Input: dimensioned drawing with shaded views. Units: mm. Origin: part minimum x, y, z. Give positions to 0.01 mm unless a question says otherwise; leave off trailing zeros. Order: outer loops, then holes, each group sorted by start corner. A loop starts at its lowest first (then second) coordinate and runs counter-clockwise, first axis right, second up. Notation, with made-up numbers: (22.5, 11) -> (79.5, 11) arc R15 ccw to (79.5, 15) -> close; hole circle Ø10 at (62.25, 55). An arc over 180 degrees is marked (long way). Use CSV: the item, a comma, the result in double quotes.
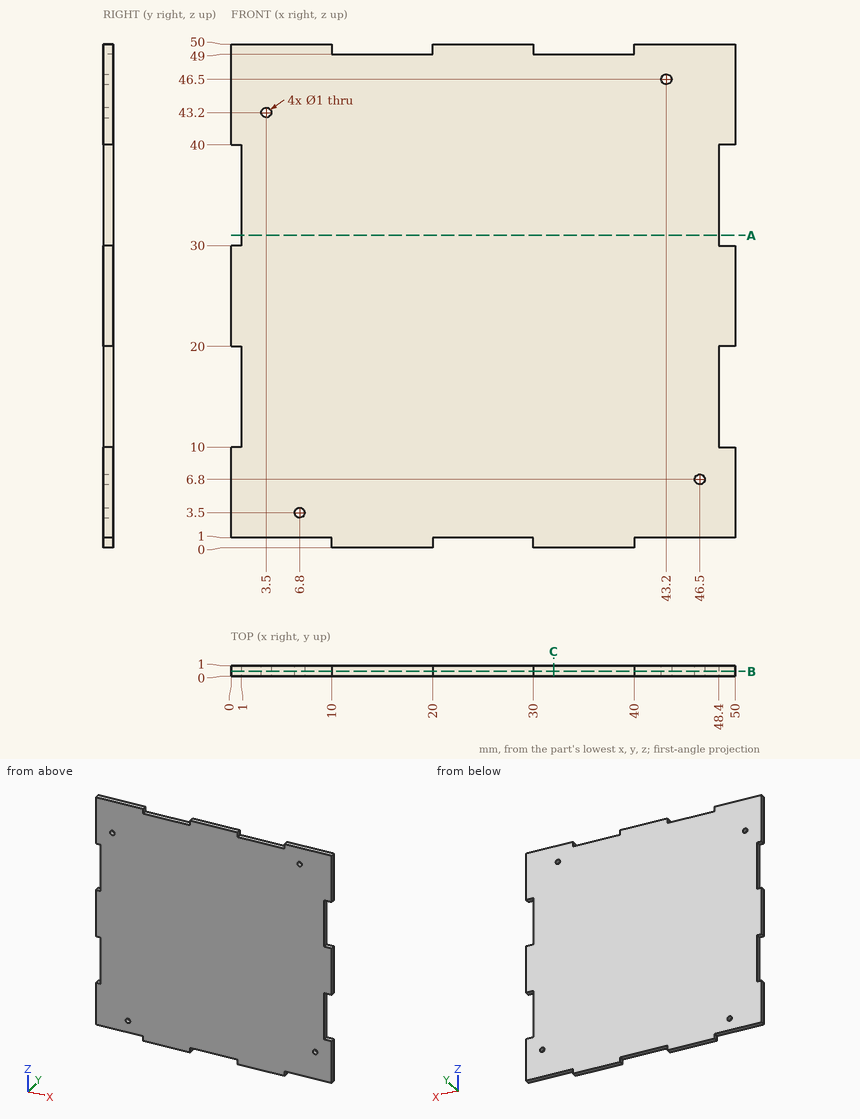
1. Section query A-A on z = 31. Return loops of the section in (x, y), plus the area to 3 significant figures.
Answer below:
outline,"(1, 0) -> (48.4, 0) -> (48.4, 1) -> (1, 1) -> close"
area,"47.4 mm²"
2. Section query B-B on y = 0.45. Count the separate pieces of the cut face and the enclosed holes in it, plus the area to 3 significant figures.
Answer below:
separate pieces,"1"
enclosed holes,"4"
area,"2,390 mm²"
3. Section query C-C on x = 32. Return loops of the section in (y, z).
Answer below:
outline,"(0, 0) -> (1, 0) -> (1, 49) -> (0, 49) -> close"
4. Pin query (flat end, axial travel): P1, Ø0.5, axis at x = 6.5, y = 0.5, coming from the -Z side; P2, Ø0.5, axis at y = 0.5, z = 0.5, coming from the -X side. Return the tip coordinate at first contact, or that it passes through.
Answer below:
P1,"stops at z = 1"
P2,"stops at x = 10"
5. Ray query, line 1 along Z through (x, y) = (43.2, 0.6); line 2 along Z through (x, y) = (46.5, 0.4); line 3 along X through (y, z) = (0.6, 3.5). Return the intervals inside material, ascending.
Answer below:
line 1,"z = 1 to 46, 47 to 50"
line 2,"z = 1 to 6.3, 7.3 to 50"
line 3,"x = 0 to 6.3, 7.3 to 50"
